Build history of the part. All positions in model axes, mm. A direction names the side the tool comes from. Give positions to 0.01 mm unless a question says otherwise; leave off trailing zeros. Use a Markdown table: item, result. Add a question column.
(1) Which spindle directions (+Z, -Z, +X, -X, +Y, -Y) get a long thin tool onto all of the face, cutting with end or side? Do faces 4 (the face through (-3, 12, 0)), 5 (the face through (-26.57, 6.77, 2.99)), 6 (the face through (25.18, -6.41, 5.4)), 7 (the face through (25.45, 6.62, 0.6)). Say none if no direction does.
(2) Flat gauge pins, fed straight in: pin 1 (1.5 mm diameter, centred on x = -23.5, z = 1.5, fed in from +Y); pin 2 (6 mm diameter, centred on x = 7.5, y = -33.5, fed in from +Z); pin 3 (3 mm diameter, centred on x = -33.5, y = 13, fed in from -Z); pin 4 (5 mm diameter, centred on x = 33, y = -29, fed in from -Z). Where does each tip first touch, or does it go through?
(3) Slice it at A-A (y = 2.5). Count the separate pieces of the cut face and the enclosed holes in it, then the cut area to 3 significant figures.
(4) Mould opens along Y. For faces 1 (the face through (25.18, -6.41, 0.6)), 2 (the face through (-3, 12, 6)), 3 (the face through (26.57, -6.77, 2.99)) say: +Y half, -Y half, draft (parallel to the pull), parting line (faces both ways), or undercut.
(5) Wall check: line 1 (X direction, y = -12.5, z = 2.25); line 2 (X direction, y = -28, z = 4.25); line 3 (X direction, y = 19.5, z = 1). Give the ranges that are in metal, low to high.
from build123d import *

# Parameters (mm, degrees)
F0_R     = 11
F1_DEPTH = 6
F2_R     = 2


with BuildPart() as f1:
    # F0 (on Top) → F1 (new body)
    with BuildSketch(Plane.XY):
        with BuildLine():
            Line((0, -17.9097384963), (13.3603457361, -35))
            ThreePointArc((13.3603457361, -35), (16.6545076898, -33.5578040372), (19.7952198288, -31.8064161785))
            ThreePointArc((19.7952198288, -31.8064161785), (13.0796897832, -13.0796897832), (31.8064161785, -19.7952198288))
            ThreePointArc((31.8064161785, -19.7952198288), (33.5578040372, -16.6545076898), (35, -13.3603457361))
            Line((35, -13.3603457361), (17.9097384963, 0))
            Line((17.9097384963, 0), (35, 13.3603457361))
            ThreePointArc((35, 13.3603457361), (33.5578040372, 16.6545076898), (31.8064161785, 19.7952198288))
            ThreePointArc((31.8064161785, 19.7952198288), (13.0796897832, 13.0796897832), (19.7952198288, 31.8064161785))
            ThreePointArc((19.7952198288, 31.8064161785), (16.6545076898, 33.5578040372), (13.3603457361, 35))
            Line((13.3603457361, 35), (0, 17.9097384963))
            Line((0, 17.9097384963), (-13.3603457361, 35))
            ThreePointArc((-13.3603457361, 35), (-16.6545076898, 33.5578040372), (-19.7952198288, 31.8064161785))
            ThreePointArc((-19.7952198288, 31.8064161785), (-12.712648295, 28.2507971495), (-9.8578643763, 20.8578643763))
            ThreePointArc((-9.8578643763, 20.8578643763), (-20.3259197477, 9.8707339542), (-31.8064161785, 19.7952198288))
            ThreePointArc((-31.8064161785, 19.7952198288), (-33.5578040372, 16.6545076898), (-35, 13.3603457361))
            Line((-35, 13.3603457361), (-17.9097384963, 0))
            Line((-17.9097384963, 0), (-35, -13.3603457361))
            ThreePointArc((-35, -13.3603457361), (-33.5578040372, -16.6545076898), (-31.8064161785, -19.7952198288))
            ThreePointArc((-31.8064161785, -19.7952198288), (-20.3259197477, -9.8707339542), (-9.8578643763, -20.8578643763))
            ThreePointArc((-9.8578643763, -20.8578643763), (-12.712648295, -28.2507971495), (-19.7952198288, -31.8064161785))
            ThreePointArc((-19.7952198288, -31.8064161785), (-16.6545076898, -33.5578040372), (-13.3603457361, -35))
            Line((-13.3603457361, -35), (0, -17.9097384963))
        make_face()
        Circle(F0_R, mode=Mode.SUBTRACT)
        with BuildLine():
            ThreePointArc((-24.1091269025, 35), (-30.0520382004, 30.0520382004), (-35, 24.1091269025))
            Line((-35, 24.1091269025), (-35, 13.3603457361))
            ThreePointArc((-35, 13.3603457361), (-33.5578040372, 16.6545076898), (-31.8064161785, 19.7952198288))
            ThreePointArc((-31.8064161785, 19.7952198288), (-28.6360389693, 28.6360389693), (-19.7952198288, 31.8064161785))
            ThreePointArc((-19.7952198288, 31.8064161785), (-16.6545076898, 33.5578040372), (-13.3603457361, 35))
            Line((-13.3603457361, 35), (-24.1091269025, 35))
        make_face()
        with BuildLine():
            ThreePointArc((24.1091269025, 35), (0, 42.5), (-24.1091269025, 35))
            Line((-24.1091269025, 35), (-13.3603457361, 35))
            ThreePointArc((-13.3603457361, 35), (0, 37.4632998839), (13.3603457361, 35))
            Line((13.3603457361, 35), (24.1091269025, 35))
        make_face()
        with BuildLine():
            ThreePointArc((31.8064161785, 19.7952198288), (33.5578040372, 16.6545076898), (35, 13.3603457361))
            Line((35, 13.3603457361), (35, 24.1091269025))
            ThreePointArc((35, 24.1091269025), (30.0520382004, 30.0520382004), (24.1091269025, 35))
            Line((24.1091269025, 35), (13.3603457361, 35))
            ThreePointArc((13.3603457361, 35), (16.6545076898, 33.5578040372), (19.7952198288, 31.8064161785))
            ThreePointArc((19.7952198288, 31.8064161785), (28.2507971495, 29.0030804576), (31.8578643763, 20.8578643763))
            ThreePointArc((31.8578643763, 20.8578643763), (31.8449947984, 20.3259197477), (31.8064161785, 19.7952198288))
        make_face()
        with BuildLine():
            Line((35, -13.3603457361), (35, -24.1091269025))
            ThreePointArc((35, -24.1091269025), (40.5817077019, -12.624381173), (42.5, 0))
            ThreePointArc((42.5, 0), (40.5817077019, 12.624381173), (35, 24.1091269025))
            Line((35, 24.1091269025), (35, 13.3603457361))
            ThreePointArc((35, 13.3603457361), (36.8423284696, 6.792766088), (37.4632998839, 0))
            ThreePointArc((37.4632998839, 0), (36.8423284696, -6.792766088), (35, -13.3603457361))
        make_face()
        with BuildLine():
            ThreePointArc((19.7952198288, -31.8064161785), (16.6545076898, -33.5578040372), (13.3603457361, -35))
            Line((13.3603457361, -35), (24.1091269025, -35))
            ThreePointArc((24.1091269025, -35), (30.0520382004, -30.0520382004), (35, -24.1091269025))
            Line((35, -24.1091269025), (35, -13.3603457361))
            ThreePointArc((35, -13.3603457361), (33.5578040372, -16.6545076898), (31.8064161785, -19.7952198288))
            ThreePointArc((31.8064161785, -19.7952198288), (31.8449947984, -20.3259197477), (31.8578643763, -20.8578643763))
            ThreePointArc((31.8578643763, -20.8578643763), (28.2507971495, -29.0030804576), (19.7952198288, -31.8064161785))
        make_face()
        with BuildLine():
            Line((24.1091269025, -35), (13.3603457361, -35))
            ThreePointArc((13.3603457361, -35), (0, -37.4632998839), (-13.3603457361, -35))
            Line((-13.3603457361, -35), (-24.1091269025, -35))
            ThreePointArc((-24.1091269025, -35), (0, -42.5), (24.1091269025, -35))
        make_face()
        with BuildLine():
            Line((-24.1091269025, -35), (-13.3603457361, -35))
            ThreePointArc((-13.3603457361, -35), (-16.6545076898, -33.5578040372), (-19.7952198288, -31.8064161785))
            ThreePointArc((-19.7952198288, -31.8064161785), (-28.6360389693, -28.6360389693), (-31.8064161785, -19.7952198288))
            ThreePointArc((-31.8064161785, -19.7952198288), (-33.5578040372, -16.6545076898), (-35, -13.3603457361))
            Line((-35, -13.3603457361), (-35, -24.1091269025))
            ThreePointArc((-35, -24.1091269025), (-30.0520382004, -30.0520382004), (-24.1091269025, -35))
        make_face()
        with BuildLine():
            ThreePointArc((-35, 24.1091269025), (-42.5, 0), (-35, -24.1091269025))
            Line((-35, -24.1091269025), (-35, -13.3603457361))
            ThreePointArc((-35, -13.3603457361), (-37.4632998839, 0), (-35, 13.3603457361))
            Line((-35, 13.3603457361), (-35, 24.1091269025))
        make_face()
    extrude(amount=F1_DEPTH)

    # F2
    f2_edges = [f1.edges().sort_by_distance(p)[0] for p in [
        (35, -24.109127, 6),
        (35, -24.109127, 0),
        (-26.454869, 6.680173, 6),
        (-26.454869, -6.680173, 6),
        (-6.680173, -26.454869, 6),
        (6.680173, -26.454869, 6),
        (26.454869, -6.680173, 6),
        (26.454869, 6.680173, 6),
        (6.680173, 26.454869, 6),
        (-6.680173, 26.454869, 6),
        (6.680173, 26.454869, 0),
        (-6.680173, 26.454869, 0),
        (-26.454869, 6.680173, 0),
        (-26.454869, -6.680173, 0),
        (-6.680173, -26.454869, 0),
        (6.680173, -26.454869, 0),
        (26.454869, -6.680173, 0),
        (26.454869, 6.680173, 0),
    ]]
    fillet(f2_edges, radius=F2_R)


solid = f1.part
Solution:
| question | item | result |
|---|---|---|
| 1 | face 4 | -Z, +X, -X, +Y, -Y |
| 1 | face 5 | +Z, -Z |
| 1 | face 6 | +Z |
| 1 | face 7 | -Z |
| 2 | pin 1 | y = 35.85 |
| 2 | pin 2 | through |
| 2 | pin 3 | z = 0 |
| 2 | pin 4 | z = 0.23 |
| 3 | separate pieces | 4 |
| 3 | enclosed holes | 0 |
| 3 | area | 176 mm2 |
| 4 | face 1 | undercut |
| 4 | face 2 | draft |
| 4 | face 3 | undercut |
| 5 | line 1 | -40.62 to -35.32, -33.9 to -28.01, -13.71 to 13.71, 28.01 to 33.9, 35.32 to 40.62 |
| 5 | line 2 | -31.95 to -29.22, -12.49 to -7.91, 7.91 to 12.49, 29.22 to 31.95 |
| 5 | line 3 | -37.46 to -31.77, -9.94 to -1.58, 1.58 to 9.94, 31.77 to 37.46 |
